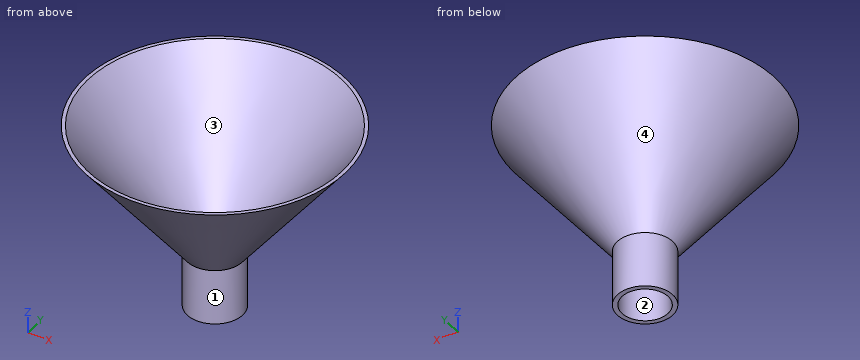
from build123d import *

# Parameters (mm, degrees)
F2_R     = 10.571716
F3_DEPTH = 22.86
F4_R     = 10.571716
F5_DEPTH = 25.4


with BuildPart() as f1:
    # F0 (on Front) → F1 (revolve)
    with BuildSketch(Plane.XZ):
        Polygon((8.974869, -30.552745), (21.674869, -30.552745), (21.674869, -5.152745), (68.532457, 54.937241), (66.91015, 54.937241), (24.070622, 0), (8.974869, 0), align=None)
    revolve(axis=Axis((8.974869, 0, -15.276372), (0, 0, 1)))

    # F2 (on face) → F3 (cut)
    with BuildSketch(Plane(origin=(0, 0, -30.552745), x_dir=(1, 0, 0), z_dir=(0, 0, -1))):
        with Locations((8.974869, 0)):
            Circle(F2_R)
    extrude(amount=-F3_DEPTH, mode=Mode.SUBTRACT)

    # F4 (on face) → F5 (cut)
    with BuildSketch(Plane(origin=(0, 0, -7.692745), x_dir=(1, 0, 0), z_dir=(0, 0, -1))):
        with Locations((8.974869, 0)):
            Circle(F4_R)
    extrude(amount=-F5_DEPTH, mode=Mode.SUBTRACT)


solid = f1.part
Geometry: final body of the model. Coordinates: model frame, mm. Face numbers are marked on the shaded views. A direction names the side the tool comes from. Coordinates: 2 decimals unless noted, no trailing zeros. Order: outer loops, then holes, each group sorted by start corner. A loop starts at its lowest first (then second) coordinate and runs counter-clockwise, first axis right, second up.
(1) Draft query along X for the marked faces 3 and 4. Return one class per face: pulls with the +X half, pulls with the -X half, needs draft (parallel to the pull), parting line crosses it, or undercut.
(2) Material intervals for probe 1 along Y at (x, z) = (56.5, 48); probe 2 along X at (y, z) = (13, 24); probe 3 along X at (y, z) = (9, 23.5), sorted ascending.
(3) Access query for the marked faces 1 and 2. Directions: +Z, -Z, +X, -X, +Y, -Y. A direction counts if a zero-diameter tool reaches every point of the face in a straight line with its end or side. Return the directions, or none.
(4) Section query A-A (y = 0). Return the cut outline in (x, z).
(5) First-contact query: pin 1 (10 mm diameter, centred on x = 2, z = -22, fed in from +Y); pin 2 (2 mm diameter, centred on x = 8.5, z = -3.5, fed in from +Y); pin 3 (1.5 mm diameter, centred on x = -10.5, z = 46, fed in from +Y). Flat tips, straight axial feed; report the tip coordinate or a pass-through.
(6) Section query C-C (z = 17). Return the cut outline in (x, y), plus the area to 3 significant figures.
(7) Section query B-B (z = 38.5). Return the cut outline in (x, y).
Solution:
1. face 3: undercut
1. face 4: parting line crosses it
2. probe 1: y = -25.95 to -22.37, 22.37 to 25.95
2. probe 2: x = -23.99 to -22.24, 40.19 to 41.94
2. probe 3: x = -24.89 to -23.21, 41.16 to 42.84
3. face 1: -Z
3. face 2: +Z, -Z
4. outline: (-50.58, 54.94) - (-3.73, -5.15) - (-3.73, -30.55) - (-1.6, -30.55) - (-1.6, 0) - (-6.12, 0) - (-48.96, 54.94) - close; (19.55, -30.55) - (21.67, -30.55) - (21.67, -5.15) - (68.53, 54.94) - (66.91, 54.94) - (24.07, 0) - (19.55, 0) - close
5. pin 1: stops at y = 12.55
5. pin 2: stops at y = 14.76
5. pin 3: stops at y = 49.54
6. outline: circle Ø59.95 at (8.97, 0); hole circle Ø56.7 at (8.97, 0)
6. area: 297 mm2
7. outline: circle Ø93.48 at (8.97, 0); hole circle Ø90.24 at (8.97, 0)
